from build123d import *

# Parameters (mm, degrees)
BOSS_EXTRUDE1_DEPTH     = 220
F_20_0MM_DOWEL_HOLE1_D  = 20
FILLET1_R               = 75
SKETCH4_R               = 75
CUT_EXTRUDE1_DEPTH      = 458.263600126
F_8_0_MM_DOWEL_HOLES1_D = 8.3


with BuildPart() as part:
    # Sketch1 → Boss-Extrude1 (new body)
    with BuildSketch(Plane.XY):
        Polygon((-4, 393), (-4, 8), (-75, 8), (-75, 0), (75, 0), (75, 8), (4, 8), (4, 393), align=None)
    extrude(amount=BOSS_EXTRUDE1_DEPTH)

    # Ø20.0mm Dowel Hole1 (through all)
    with Locations(Plane(origin=(0, 0, 0), x_dir=(-1, 0, 0), z_dir=(0, -1, 0))):
        with Locations((-40, -55), (-40, -165), (40, -165), (40, -55)):
            Hole(F_20_0MM_DOWEL_HOLE1_D / 2)

    # Fillet1
    fillet1_edges = [part.edges().sort_by_distance(p)[0] for p in [
        (0, 393, 0),
        (0, 393, 220),
    ]]
    fillet(fillet1_edges, radius=FILLET1_R)

    # Sketch4 → Cut-Extrude1 (cut, through all)
    with BuildSketch(Plane(origin=(4, 0, 0), x_dir=(0, 0, -1), z_dir=(1, 0, 0))):
        with Locations(Location((-110, 283, 0), (0, 0, 90))):
            Circle(SKETCH4_R)
    extrude(amount=-CUT_EXTRUDE1_DEPTH, mode=Mode.SUBTRACT)

    # Ø8.0 mm Dowel Holes1 (through all)
    with Locations(Plane(origin=(4, 0, 0), x_dir=(0, 0, -1), z_dir=(1, 0, 0))):
        with Locations((-110, 368), (-195, 283), (-110, 198), (-25, 283)):
            Hole(F_8_0_MM_DOWEL_HOLES1_D / 2)


solid = part.part
Read the model definition and answer for the solid it produces. Units are mm, in the model's axes. A direction names the side the tool comes from. Coordinates: 2 decimals unless noted, no trailing zeros. Loops run counter-clockwise (first coordinate to the right, second up) from the corner with the lowest first, then second, coordinate; pieces in that order, holes last. Notation, with made-up numbers: (78, 81) -> (110, 81) arc R27 ccw to (110, 98) -> close; hole circle Ø9 at (49, 43.25). An arc over 180 degrees is marked (long way). Write item = value, one per line. Start each with the question number.
1) Find the intervals of material crossed by L1, parallel to X at y = 4, z = 165; L2, parallel to Z at x = -1.75, y = 283; L3, parallel to Z at x = 40, y = 4.5, in increasing order. Write a range as from..to.
2) The part is cut by section C-C, the plane y = 283. Determine the outline of the cut face in (x, z), plus the area to 3 significant figures.
3) For faces 1 (the face through (4, 155, 108)), 2 (the face through (-0.06, 371.61, 197.45)), 3 (the face through (-39, 8, 108)), determine the directions among +Z, -Z, +X, -X, +Y, -Y from which every point of the face is accessible in a straight line to the end or side of a thin tool.
4) The part is cut by section B-B, the plane x = 40. Determine the outline of the cut face in (y, z), plus the area to 3 significant figures.
5) The mould has two halves that part along Y. Classify faces 4 (the face through (0, 89, 0)), 5 (the face through (-0.06, 278.95, 194.1)), 6 (the face through (40, 8, 108)): pulls with the +Y half, pulls with the -Y half, needs draft (parallel to the pull), parting line crosses it, or undercut.
6) The part is cut by section A-A, the plane y = 198. Determine the outline of the cut face in (x, z), plus the area to 3 significant figures.
7) Given P1, Ø5, axis at y = 198.5, z = 90.5, coming from the -X side; P2, Ø6.5, axis at y = 283, z = 25, coming from the +X side; P3, Ø10, axis at x = -58.5, z = 78, coming from the -Y side; P4, Ø21.5, axis at x = 47, z = 141, coming from the +Y side, each flat-ended and moving along its own axis, determine where each tip first touches the part or whether it passes through.
8) The part is cut by section D-D, the plane z = 195. Determine the outline of the cut face in (x, y).
Result:
q1.L1 = -75..-50, -30..30, 50..75
q1.L2 = 0..20.85, 29.15..35, 185..190.85, 199.15..220
q1.L3 = 0..45, 65..155, 175..220
q2.outline = (-4, 0) -> (4, 0) -> (4, 20.85) -> (-4, 20.85) -> close; (-4, 29.15) -> (4, 29.15) -> (4, 35) -> (-4, 35) -> close; (-4, 185) -> (4, 185) -> (4, 190.85) -> (-4, 190.85) -> close; (-4, 199.15) -> (4, 199.15) -> (4, 220) -> (-4, 220) -> close
q2.area = 427 mm²
q3.face_1 = +Z, -Z, +X, +Y
q3.face_2 = +Z, +X, -X, +Y
q3.face_3 = +Z, -Z, -X, +Y
q4.outline = (0, 0) -> (8, 0) -> (8, 45) -> (0, 45) -> close; (0, 65) -> (8, 65) -> (8, 155) -> (0, 155) -> close; (0, 175) -> (8, 175) -> (8, 220) -> (0, 220) -> close
q4.area = 1,440 mm²
q5.face_4 = needs draft
q5.face_5 = undercut
q5.face_6 = pulls with the +Y half
q6.outline = (-4, 0) -> (4, 0) -> (4, 105.85) -> (-4, 105.85) -> close; (-4, 114.15) -> (4, 114.15) -> (4, 220) -> (-4, 220) -> close
q6.area = 1,690 mm²
q7.P1 = -4
q7.P2 = through
q7.P3 = 0
q7.P4 = 8
q8.outline = (-75, 0) -> (75, 0) -> (75, 8) -> (4, 8) -> (4, 278.85) -> (-4, 278.85) -> (-4, 8) -> (-75, 8) -> close; (-4, 287.15) -> (4, 287.15) -> (4, 373.9) -> (-4, 373.9) -> close
